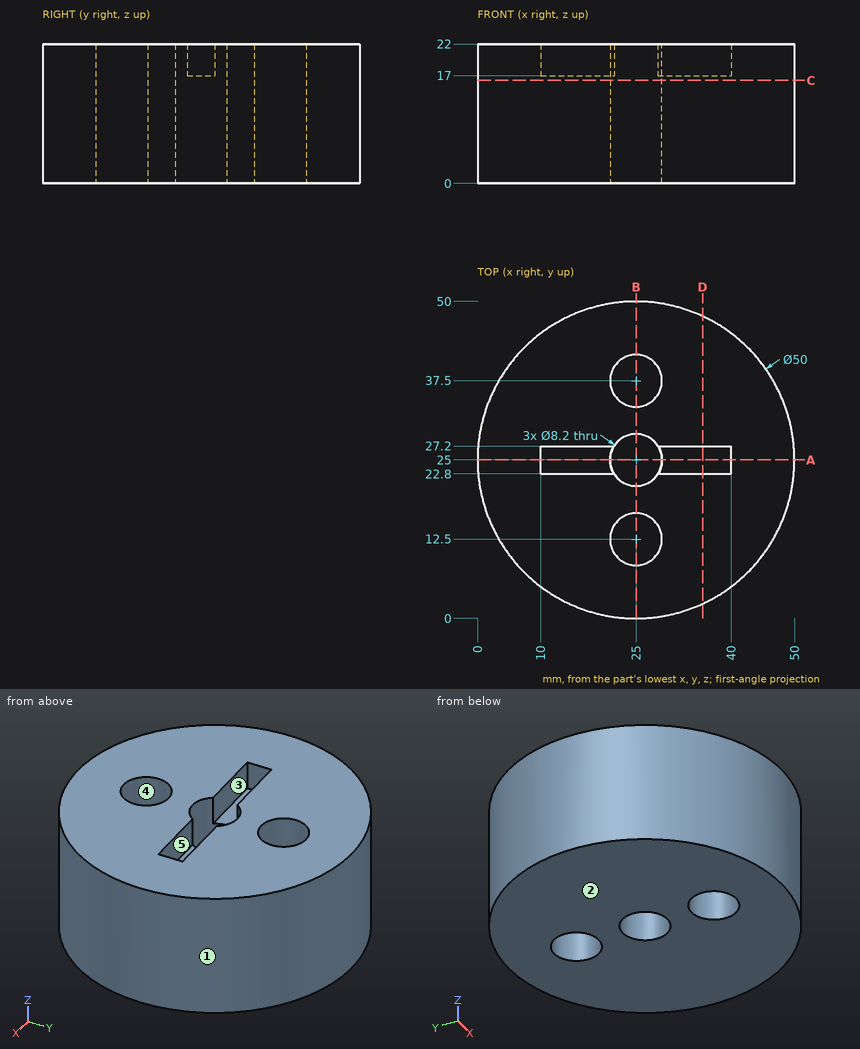
Job drawing, mm, ordinate dimensions from the low corner. One solid piece. A direction names the side the tool comes from. Give positions to 0.01 mm unless a question says otherwise; leave off trailing zeros. Write each loop counter-clockwise with the first axis right and the second up, starting at its lowest first coordinate (ties: lowest second). Pieces come first, ordered by that corner, then holes. Notation, with made-up numbers: M 12.25,49 L 70.25,49 A26 ccw 70.25,83 Z; hole C 59.5,-5.5 d5. An arc over 180 degrees is marked long. One line per item, written item: value. Start each with the question number.
Q1. Saw through at D-D, the plane x = 35.5. Write the cut outline in (y, z), plus the area to 3 significant figures.
Q2. Probe probe 1 along Y at (x, z) = (25, 16.25); probe 2 along X at (y, z) = (41, 11.25); probe 3 along Y at (x, z) = (22.5, 1.75). List the from-to ranges inside material, lowest first. Write a range as [from, to].
Q3. 3-axis set-ups, long thin cutter, end or side, ignore diameter. For the marked faces 4 and 5: which of +Z, -Z, +X, -X, +Y, -Y reach the whole face in a straight line?
Q4. Two-plate mould, pull along Y, no slides. Class the marked faces 1, 2 and 3: +Y half, -Y half, draft (parallel to the pull), parting line (faces both ways), or undercut.
Q5. Saw through at B-B, the plane x = 25. Write the cut outline in (y, z).
Q6. Drop flat-ended pins along their axis: pin 1 Ø2.5 at (x, z) = (31.5, 19) entering from -Y; pin 2 Ø1.5 at (x, z) = (13, 18.5) entering from -Y; pin 3 Ø1 at (x, z) = (34.5, 11.5) entering from -Y; pin 4 Ø3 at (x, y) = (27, 26) entering from +Z. Give the stop position or say it passes through.
Q7. Saw through at C-C, the plane z = 16.25. Write the cut outline in (x, y).
Q8. Saw through at A-A, the plane y = 25. Write the cut outline in (x, z), plus the area to 3 significant figures.
Output values:
1. outline: M 2.31,0 L 47.69,0 L 47.69,22 L 27.2,22 L 27.2,17 L 22.8,17 L 22.8,22 L 2.31,22 Z
1. area: 976 mm²
2. probe 1: y = [0, 8.4], [16.6, 20.9], [29.1, 33.4], [41.6, 50]
2. probe 2: x = [5.79, 22.86], [27.14, 44.21]
2. probe 3: y = [0.13, 9.25], [15.75, 21.75], [28.25, 34.25], [40.75, 49.87]
3. face 4: +Z, -Z
3. face 5: +Z
4. face 1: parting line
4. face 2: draft
4. face 3: undercut
5. outline: M 0,0 L 8.4,0 L 8.4,22 L 0,22 Z; M 16.6,0 L 20.9,0 L 20.9,22 L 16.6,22 Z; M 29.1,0 L 33.4,0 L 33.4,22 L 29.1,22 Z; M 41.6,0 L 50,0 L 50,22 L 41.6,22 Z
6. pin 1: stops at y = 0.56
6. pin 2: stops at y = 2.67
6. pin 3: stops at y = 1.68
6. pin 4: passes through
7. outline: C 25,25 d50; hole C 25,12.5 d8.2; hole C 25,25 d8.2; hole C 25,37.5 d8.2
8. outline: M 0,0 L 20.9,0 L 20.9,17 L 10,17 L 10,22 L 0,22 Z; M 29.1,0 L 50,0 L 50,22 L 40,22 L 40,17 L 29.1,17 Z
8. area: 811 mm²
